Could you check a few things on this model? Use its own coordinates, in mm. A direction names the side the tool comes from. Give positions to 0.01 mm unless a question says otherwise; leave off trailing zeros. Loops run counter-clockwise (first coordinate to the right, second up) from the corner with the lowest first, then second, coordinate; pieces in that order, holes last. Notation, with made-up numbers: (-3, 68.5) -> (38, 68.5) arc R20 cw to (38, 79.5) -> close; hole circle Ø9 at (75.25, 25.5). An arc over 180 degrees is marked (long way). Write item = value, one per line. Start each with the question number.
1) I want a section at B-B (x = 37). List the corners of the cut face in (y, z) for me (3 decimals).
2) I'm going to push flat-ended pins straight in: pin 1 Ø2 at (x, y) = (14, -19) entering from -Z; pin 2 Ø1.5 at (x, y) = (102, 0) entering from +Z. Where does each tip first touch, or does it pass through?
3) If we mould it in two halves opening along X, with no side actions, what happens to faces 1 (the face through (50, -27.3, 0)), 2 (the face through (98.615, -0.751, -0.764)), 3 (the face through (93.198, -0.523, -1.976))? For each: +X half, -X half, draft (parallel to the pull), parting line (faces both ways), or undercut.
4) I need wall thicknesses on probe 1 along Z at (x, y) = (-41, -7); probe 2 along X at (y, z) = (-16, -1.6); probe 3 along X at (y, z) = (18, -0.8). Which ranges of each line are inside material? Lowest first, please. Write a range as from..to.
5) I want a section at C-C (y = -22.8). Count the separate pieces of the cut face and the enclosed holes in it, and give its area (3 significant figures).
6) I want a section at D-D (x = 101). List the corners of the cut face in (y, z) for me (3 decimals).
7) On a 3-axis mill with a long thin cutter (end or side, diameter ignored), from which of +Z, -Z, +X, -X, +Y, -Y can I reach the whole of each face in a straight line? I mean faces 4 (the face through (101, -8, -1.75)), 5 (the face through (34.61, 19.55, 0)). Say none if no direction works.
8) I want a section at A-A (y = 0). List the corners of the cut face in (x, z) for me.
from build123d import *

# Parameters (mm, degrees)
SKETCH1_W               = 250
SKETCH1_H               = 100
BOSS_EXTRUDE1_DEPTH     = 0.25
SKETCH2_R               = 2.4
CUT_EXTRUDE1_DEPTH      = 135.630048652
SKETCH3_W               = 375
SKETCH3_H               = 252.815
SKETCH3_W_2             = 175
SKETCH3_H_2             = 52.815
CUT_EXTRUDE_THIN1_DEPTH = 135.630048652
SKETCH6_W               = 8
SKETCH6_H               = 52.815
BOSS_EXTRUDE3_DEPTH     = 3.5
CUT_EXTRUDE2_DEPTH      = 109.564681181
CUT_EXTRUDE2_DEPTH_BACK = 2
SKETCH5_R               = 2.5
BOSS_EXTRUDE4_DEPTH     = 52.815


with BuildPart() as part:
    # Sketch1 → Boss-Extrude1 (new, symmetric)
    with BuildSketch(Plane.XY):
        Rectangle(SKETCH1_W, SKETCH1_H)
    extrude(amount=BOSS_EXTRUDE1_DEPTH, both=True)

    # Sketch2 → Cut-Extrude1 (cut, through all)
    with BuildSketch(Plane.XY.offset(0.25)):
        with Locations((-51.1175, -22.8)):
            Circle(SKETCH2_R)
        with Locations((-36.5125, -22.8)):
            Circle(SKETCH2_R)
        with Locations((-21.9075, -22.8)):
            Circle(SKETCH2_R)
        with Locations((-7.3025, -22.8)):
            Circle(SKETCH2_R)
        with Locations((7.3025, -22.8)):
            Circle(SKETCH2_R)
        with Locations((21.9075, -22.8)):
            Circle(SKETCH2_R)
        with Locations((36.5125, -22.8)):
            Circle(SKETCH2_R)
        with Locations((51.1175, -22.8)):
            Circle(SKETCH2_R)
        with Locations((-36.5125, -8.195)):
            Circle(SKETCH2_R)
        with Locations((-21.9075, -8.195)):
            Circle(SKETCH2_R)
        with Locations((-7.3025, -8.195)):
            Circle(SKETCH2_R)
        with Locations((7.3025, -8.195)):
            Circle(SKETCH2_R)
        with Locations((21.9075, -8.195)):
            Circle(SKETCH2_R)
        with Locations((36.5125, -8.195)):
            Circle(SKETCH2_R)
        with Locations((51.1175, -8.195)):
            Circle(SKETCH2_R)
        with Locations((-36.5125, 6.41)):
            Circle(SKETCH2_R)
        with Locations((-21.9075, 6.41)):
            Circle(SKETCH2_R)
        with Locations((-7.3025, 6.41)):
            Circle(SKETCH2_R)
        with Locations((7.3025, 6.41)):
            Circle(SKETCH2_R)
        with Locations((21.9075, 6.41)):
            Circle(SKETCH2_R)
        with Locations((36.5125, 6.41)):
            Circle(SKETCH2_R)
        with Locations((51.1175, 6.41)):
            Circle(SKETCH2_R)
        with Locations((-36.5125, 21.015)):
            Circle(SKETCH2_R)
        with Locations((-21.9075, 21.015)):
            Circle(SKETCH2_R)
        with Locations((-7.3025, 21.015)):
            Circle(SKETCH2_R)
        with Locations((7.3025, 21.015)):
            Circle(SKETCH2_R)
        with Locations((21.9075, 21.015)):
            Circle(SKETCH2_R)
        with Locations((36.5125, 21.015)):
            Circle(SKETCH2_R)
        with Locations((51.1175, 21.015)):
            Circle(SKETCH2_R)
        with Locations((-51.1175, -8.195)):
            Circle(SKETCH2_R)
        with Locations((-51.1175, 6.41)):
            Circle(SKETCH2_R)
        with Locations((-51.1175, 21.015)):
            Circle(SKETCH2_R)
    extrude(amount=-CUT_EXTRUDE1_DEPTH, mode=Mode.SUBTRACT)

    # Sketch3 → Cut-Extrude-Thin1 (cut, through all)
    with BuildSketch(Plane.XY.offset(0.25)):
        with Locations((17.5, -0.8925)):
            Rectangle(SKETCH3_W, SKETCH3_H)
        with Locations((17.5, -0.8925)):
            Rectangle(SKETCH3_W_2, SKETCH3_H_2, mode=Mode.SUBTRACT)
    extrude(amount=-CUT_EXTRUDE_THIN1_DEPTH, mode=Mode.SUBTRACT)

    # Sketch6 → Boss-Extrude3 (add)
    with BuildSketch(Plane(origin=(0, 0, -0.25), x_dir=(-1, 0, 0), z_dir=(0, 0, -1))):
        with Locations((-101, -0.8925)):
            Rectangle(SKETCH6_W, SKETCH6_H)
    extrude(amount=BOSS_EXTRUDE3_DEPTH)

    # Sketch5 → Cut-Extrude2 (cut, two sides: drawn at the far end of the back side and taken through both)
    with BuildSketch(Plane.XY.offset(0.25).offset(-CUT_EXTRUDE2_DEPTH_BACK)):
        with Locations(Location((101, -16, 0), (0, 0, 180))):
            Circle(SKETCH5_R)
        with Locations(Location((101, -8, 0), (0, 0, 180))):
            Circle(SKETCH5_R)
        with Locations(Location((101, 0, 0), (0, 0, 180))):
            Circle(SKETCH5_R)
        with Locations(Location((101, 8, 0), (0, 0, 180))):
            Circle(SKETCH5_R)
        with Locations(Location((101, 16, 0), (0, 0, 180))):
            Circle(SKETCH5_R)
    extrude(amount=CUT_EXTRUDE2_DEPTH + CUT_EXTRUDE2_DEPTH_BACK, mode=Mode.SUBTRACT)

    # Sketch8 → Boss-Extrude4 (add, through all)
    with BuildSketch(Plane(origin=(0, 25.515, 0), x_dir=(1, 0, 0), z_dir=(0, 1, 0))):
        Polygon((89.5, 0.25), (97, 3.75), (97, 0.25), align=None)
    extrude(amount=-BOSS_EXTRUDE4_DEPTH)


solid = part.part
Answer list:
q1.outline = (-27.3, -0.25) -> (-25.15, -0.25) -> (-25.15, 0.25) -> (-27.3, 0.25) -> close; (-20.45, -0.25) -> (-10.545, -0.25) -> (-10.545, 0.25) -> (-20.45, 0.25) -> close; (-5.845, -0.25) -> (4.06, -0.25) -> (4.06, 0.25) -> (-5.845, 0.25) -> close; (8.76, -0.25) -> (18.665, -0.25) -> (18.665, 0.25) -> (8.76, 0.25) -> close; (23.365, -0.25) -> (25.515, -0.25) -> (25.515, 0.25) -> (23.365, 0.25) -> close
q2.pin_1 = -0.25
q2.pin_2 = -1.75
q3.face_1 = draft
q3.face_2 = undercut
q3.face_3 = -X half
q4.probe_1 = -0.25..0.25
q4.probe_2 = 92.39..98.5, 103.5..105
q4.probe_3 = 90.68..99.5, 102.5..105
q5.separate_pieces = 9
q5.enclosed_holes = 0
q5.area = 109 mm^2
q6.outline = (-27.3, -3.75) -> (25.515, -3.75) -> (25.515, 0.25) -> (18.5, 0.25) -> (18.5, -1.75) -> (13.5, -1.75) -> (13.5, 0.25) -> (10.5, 0.25) -> (10.5, -1.75) -> (5.5, -1.75) -> (5.5, 0.25) -> (2.5, 0.25) -> (2.5, -1.75) -> (-2.5, -1.75) -> (-2.5, 0.25) -> (-5.5, 0.25) -> (-5.5, -1.75) -> (-10.5, -1.75) -> (-10.5, 0.25) -> (-13.5, 0.25) -> (-13.5, -1.75) -> (-18.5, -1.75) -> (-18.5, 0.25) -> (-27.3, 0.25) -> close
q7.face_4 = +Z
q7.face_5 = +Z, -Z
q8.outline = (-70, -0.25) -> (89.5, -0.25) -> (97, -3.75) -> (105, -3.75) -> (105, 0.25) -> (103.5, 0.25) -> (103.5, -1.75) -> (98.5, -1.75) -> (98.5, 0.25) -> (-70, 0.25) -> close
